```python
from build123d import *

# Parameters (mm, degrees)
F1_DEPTH = 0.762
F2_W     = 10.4317168638
F2_H     = 1.524
F3_DEPTH = 38.1


with BuildPart() as f1:
    # F0 (on Front) → F1 (new body, symmetric)
    with BuildSketch(Plane.XZ):
        Polygon((1.7629392188, 22.6165422688), (-13.3985944025, 22.6165422688), (-13.3985944025, 6.9341756906), (18.3514055975, 6.9341756906), (18.3514055975, 15.9407987012), align=None)
    extrude(amount=F1_DEPTH, both=True)

    # F2 (on face) → F3 (join)
    with BuildSketch(Plane(origin=(0, 0.762, 0), x_dir=(-1, 0, 0), z_dir=(0, 1, 0))):
        with Locations((8.1827359706, 18.0847395862)):
            Rectangle(F2_W, F2_H)
    extrude(amount=F3_DEPTH)

    # F5: F1 across plane


with BuildPart() as f1_1:
    add(f1.part)
    add(f1.part.mirror(Plane(origin=(-8.1827359706, 38.862, 18.0847395862), x_dir=(-1, 0, 0), z_dir=(0, 1, 0))))


solid = f1_1.part
```
Geometry: final body of the model. Coordinates: model frame, mm. A direction names the side the tool comes from. Coordinates: 2 decimals unless noted, no trailing zeros. Loops run counter-clockwise (first coordinate to the right, second up) from the corner with the lowest first, then second, coordinate; pieces in that order, holes last. Notation, with made-up numbers: (77, 6.25) -> (96, 6.25) arc R24 cw to (96, 20.25) -> close; hole circle Ø7 at (-28.75, -8.75). An arc over 180 degrees is marked (long way). Use a Markdown table: item, result. Add a question column.
(1) Section query D-D, the plane y = 67.5. Return loops of the section in (x, z).
(2) Section query C-C, the plane x = -9.5. Return loops of the section in (y, z), plus the area to 3 significant figures.
(3) Line query: line 1 along Y through (x, z) = (14, 9); line 2 along X through (y, z) = (31.5, 18.75); line 3 along Z through (x, y) = (-4.5, 19). Output: solid intervals per line, ascending.
(4) Section query B-B, the plane z = 11.75. Return loops of the section in (x, y), plus the area to 3 significant figures.
(5) Mould query, pull axis Y, two halves, no side actions, for faces 1 (the flat face through (2, 78.486, 15)), 2 (the flat face through (18.351, 78, 11)), 3 (the flat face through (-2.967, 39, 18)), 4 (the flat face through (2, -0.762, 15)). Classes: pulls with the +Y half, pulls with the -Y half, needs draft (parallel to the pull), parting line crosses it, or undercut.
(6) Section query A-A, the plane x = 0. Return loops of the section in (y, z).
(7) Access query for faces 5 (the flat face through (-8, 39, 18.847)), 6 (the flat face through (-8, 39, 17.323)), 7 (the flat face through (-6, 0, 22.617)). Directions: +Z, -Z, +X, -X, +Y, -Y. A direction counts if a zero-diameter tool reaches every point of the face in a straight line with its end or side. Return the directions, or none.
(8) Pin query (flat end, axial travel): pin 1 Ø5 at (x, y) = (-7, 32.5) entering from +Z; pin 2 Ø0.5 at (y, z) = (22.5, 18) entering from +X; pin 3 Ø4 at (x, z) = (12.5, 19) entering from -Y; pin 4 Ø3 at (x, y) = (-9, 27) entering from -Z. Return the tip coordinate at first contact, or that it passes through.
Answer:
| question | item | result |
|---|---|---|
| 1 | outline | (-13.4, 17.32) -> (-2.97, 17.32) -> (-2.97, 18.85) -> (-13.4, 18.85) -> close |
| 2 | outline | (-0.76, 6.93) -> (0.76, 6.93) -> (0.76, 17.32) -> (76.96, 17.32) -> (76.96, 6.93) -> (78.49, 6.93) -> (78.49, 22.62) -> (76.96, 22.62) -> (76.96, 18.85) -> (0.76, 18.85) -> (0.76, 22.62) -> (-0.76, 22.62) -> close |
| 2 | area | 164 mm^2 |
| 3 | line 1 | y = -0.76 to 0.76, 76.96 to 78.49 |
| 3 | line 2 | x = -13.4 to -2.97 |
| 3 | line 3 | z = 17.32 to 18.85 |
| 4 | outline | (-13.4, -0.76) -> (18.35, -0.76) -> (18.35, 0.76) -> (-13.4, 0.76) -> close; (-13.4, 76.96) -> (18.35, 76.96) -> (18.35, 78.49) -> (-13.4, 78.49) -> close |
| 4 | area | 96.8 mm^2 |
| 5 | face 1 | pulls with the +Y half |
| 5 | face 2 | needs draft |
| 5 | face 3 | undercut |
| 5 | face 4 | pulls with the -Y half |
| 6 | outline | (-0.76, 6.93) -> (0.76, 6.93) -> (0.76, 22.62) -> (-0.76, 22.62) -> close; (76.96, 6.93) -> (78.49, 6.93) -> (78.49, 22.62) -> (76.96, 22.62) -> close |
| 7 | face 5 | +Z, +X, -X |
| 7 | face 6 | -Z, +X, -X |
| 7 | face 7 | +Z, +X, -X, +Y, -Y |
| 8 | pin 1 | stops at z = 18.85 |
| 8 | pin 2 | stops at x = -2.97 |
| 8 | pin 3 | stops at y = -0.76 |
| 8 | pin 4 | stops at z = 17.32 |
